The model under review builds one solid part; all positions refer to its coordinate system, in mm. A direction names the side the tool comes from. Coordinates: 2 decimals unless noted, no trailing zeros. Write each loop counter-clockwise with the first axis right and the second up, starting at its lowest first coordinate (ties: lowest second). Pieces come first, ordered by that corner, then holes. Notation, with made-up numbers: M 56,7.25 L 113,7.25 A24 ccw 113,44.25 Z; hole C 16,89 d8. An arc over 180 degrees is marked long. Answer as a JSON object with one key per item and string values.
```python
from build123d import *


with BuildPart() as part:
    # Sketch1 → Revolve1 (revolve)
    with BuildSketch(Plane.XY):
        with BuildLine():
            Line((0, 0), (-10.5, 0))
            Line((-10.5, 0), (-10.5, 7.4))
            Line((-10.5, 7.4), (-9.5, 8.4))
            Line((-9.5, 8.4), (-10, 8.4))
            Line((-10, 8.4), (-10, 13.685164654))
            ThreePointArc((-10, 13.685164654), (-9.737084783, 13.807905177), (-9.45, 13.85))
            Line((-9.45, 13.85), (-7.3, 13.85))
            Line((-7.3, 13.85), (-7.3, 20.85))
            Line((-7.3, 20.85), (-11.5, 20.85))
            Line((-11.5, 20.85), (-11.5, 24.65))
            Line((-11.5, 24.65), (0, 24.65))
            Line((0, 24.65), (0, 0))
        make_face()
    revolve(axis=Axis((0, 0, 0), (0, 1, 0)))


solid = part.part
```
(1) Add section B-B on x = 0. Give the boundary of the cut face in (y, z), and give its area (3 significant figures).
Results list:
{"outline": "M 0,-10.5 L 7.4,-10.5 L 8.4,-9.5 L 8.4,-10 L 13.69,-10 A1 ccw 13.85,-9.45 L 13.85,-7.3 L 20.85,-7.3 L 20.85,-11.5 L 24.65,-11.5 L 24.65,11.5 L 20.85,11.5 L 20.85,7.3 L 13.85,7.3 L 13.85,9.45 A1 ccw 13.69,10 L 8.4,10 L 8.4,9.5 L 7.4,10.5 L 0,10.5 Z", "area": "474 mm²"}
(2) Add section A-A on z = 0. Give the boundary of the cut face in (x, y).
Results list:
{"outline": "M -11.5,20.85 L -7.3,20.85 L -7.3,13.85 L -9.45,13.85 A1 ccw -10,13.69 L -10,8.4 L -9.5,8.4 L -10.5,7.4 L -10.5,0 L 10.5,0 L 10.5,7.4 L 9.5,8.4 L 10,8.4 L 10,13.69 A1 ccw 9.45,13.85 L 7.3,13.85 L 7.3,20.85 L 11.5,20.85 L 11.5,24.65 L -11.5,24.65 Z"}
(3) For faces 5 (the face through (2.17, 11.08, -9.76)), 6 (the face through (0, 0, 0)), 7 (the face through (-10, 3.8, 3.2)), list the 3-axis set-ups (+Z, -Z, +X, -X, +Y, -Y) from which the entire face can be reached by the end or side of a thin tool; tool diameter is ignored.
Results list:
{"face 5": "none", "face 6": "+Z, -Z, +X, -X, -Y", "face 7": "-Y"}
(4) Wall thickness on line 1 along Y through (x, z) = (-1, -9.25); line 2 along Y through (x, z) = (-2.5, -9.5); line 3 along X through (y, z) = (20, -2.5): over which ranges is each line inside the solid? List them lowest first. Write a range as from..to.
Results list:
{"line 1": "0..13.85, 20.85..24.65", "line 2": "0..8.08, 8.4..13.78, 20.85..24.65", "line 3": "-6.86..6.86"}
(5) Draft analysis for pull direction Y (two halves, no side actions). For faces 1 (the face through (1.5, 22.8, 11.4)), 2 (the face through (9, 8.4, -4)), 3 (the face through (0, 20.85, -8)), 4 (the face through (0, 24.65, 0)), state which applies: released by +Y, released by -Y, zero draft, split by the parting line, or undercut.
Results list:
{"face 1": "zero draft", "face 2": "undercut", "face 3": "undercut", "face 4": "released by +Y"}
(6) Add section C-C on y = 4.75. Give the boundary of the cut face in (x, z).
Results list:
{"outline": "C 0,0 d21"}
(7) Add section D-D on y = 16.75. Give the boundary of the cut face in (x, z).
Results list:
{"outline": "C 0,0 d14.6"}
(8) For pin 1 Ø1 at (x, y) = (-8, 13) entering from -Z; pin 2 Ø10 at (x, y) = (1, 14.5) entering from -Z; pin 3 Ø1 at (x, y) = (4, 6.5) entering from -Z, all flat-tipped, find the tip position at first contact; note any pin that passes through.
Results list:
{"pin 1": "z = -6.61", "pin 2": "z = -10", "pin 3": "z = -9.9"}
